Input: part model. Units: mm. Frame: model coordinates. Face numbers are marked on the shaded views. A direction names the side the tool comes from. Coordinates: 2 decimals unless noted, no trailing zeros. Order: outer loops, then holes, each group sorted by start corner. A loop starts at its lowest first (then second) coordinate and runs counter-clockwise, first axis right, second up. Notation, with made-up numbers: (55.5, 32) -> (97.5, 32) arc R18 cw to (97.5, 54) -> close; hole circle Ø10 at (84.5, 40). An arc over 180 degrees is marked (long way). One line per item, written item: value. Start each with the question number.
from build123d import *

# Parameters (mm, degrees)
SKETCH_1_R               = 6
SKETCH_1_R_2             = 2
EXTRUDE_1_DEPTH          = 2
SKETCH_2_R               = 1
CUT_EXTRUDE_8_DEPTH      = 40.131189606
PATTERN_CIRCULAR_2_COUNT = 4


with BuildPart() as part:
    # 草图1 → 凸台-拉伸1 (new body)
    with BuildSketch(Plane.XY):
        with BuildLine():
            Line((-3.413784582, 34.772058824), (-10.729037258, 2.426470588))
            ThreePointArc((-10.729037258, 2.426470588), (0, -11), (10.729037258, 2.426470588))
            Line((10.729037258, 2.426470588), (3.413784582, 34.772058824))
            ThreePointArc((3.413784582, 34.772058824), (0, 37.5), (-3.413784582, 34.772058824))
        make_face()
        Circle(SKETCH_1_R, mode=Mode.SUBTRACT)
        with Locations((0, 34)):
            Circle(SKETCH_1_R_2, mode=Mode.SUBTRACT)
        with BuildLine():
            Line((-2.989565186, 26.25), (-3.986086914, 14.333333333))
            ThreePointArc((-3.986086914, 14.333333333), (0, 10), (3.986086914, 14.333333333))
            Line((3.986086914, 14.333333333), (2.989565186, 26.25))
            ThreePointArc((2.989565186, 26.25), (0, 29), (-2.989565186, 26.25))
        make_face(mode=Mode.SUBTRACT)
    extrude(amount=EXTRUDE_1_DEPTH)

    # 草图2 → 切除-拉伸8 (cut, through all)
    with BuildSketch(Plane.XY):
        with Locations((6.01040764, -6.01040764)):
            Circle(SKETCH_2_R)
    cut_extrude_8 = extrude(amount=CUT_EXTRUDE_8_DEPTH, mode=Mode.SUBTRACT)

    # 阵列(圆周)2: 切除-拉伸8 ×4 about axis
    pattern_circular_2_axis = Axis((0, 0, 0), (0, 0, 1))
    for i in range(1, PATTERN_CIRCULAR_2_COUNT):
        add(cut_extrude_8.rotate(pattern_circular_2_axis, i * 360 / PATTERN_CIRCULAR_2_COUNT), mode=Mode.SUBTRACT)


solid = part.part
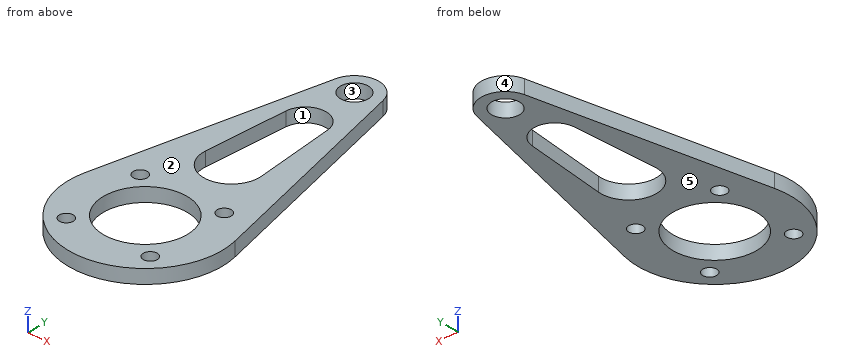
1) Pin query (flat end, axial travel): pin 1 Ø1 at (y, z) = (18, 1.5) entering from +X. Return the tip coordinate at first contact, or that it passes through.
2) Section query C-C, the plane z = 1.3. Return the cut outline in (x, y), plus the area to 3 significant figures.
3) Section query A-A, the plane x = 0. Return the cut outline in (y, z), plus the area to 3 significant figures.
4) Mould query, pull axis Y, two halves, no side actions, for the marked faces 3, 4 and 5. Classes: +Y half, -Y half, draft (parallel to the pull), parting line (faces both ways), or undercut.
5) Section query B-B, the plane y = 0. Return the cut outline in (x, z), plus the area to 3 significant figures.
6) Section query D-D, the plane x = 4.5. Return the cut outline in (y, z).
7) Ray query, line 1 along Y through (x, z) = (0.25, 0.85); line 2 along Y through (x, z) = (-1, 1.65); line 3 along X through (y, z) = (3, 1.6). Return the intervals inside material, ascending. Write a range as from..to.
8) Access query for the marked faces 1 and 2. Directions: +Z, -Z, +X, -X, +Y, -Y. A direction counts if a zero-diameter tool reaches every point of the face in a straight line with its end or side. Return the directions, or none.
Entries:
1. pin 1: stops at x = 7.32
2. outline: (-10.73, 2.43) arc R11 ccw (long way) to (10.73, 2.43) -> (3.41, 34.77) arc R3.5 ccw to (-3.41, 34.77) -> close; hole circle Ø2 at (-6.01, -6.01); hole circle Ø2 at (-6.01, 6.01); hole circle Ø12 at (0, 0); hole (-3.99, 14.33) arc R4 ccw (long way) to (3.99, 14.33) -> (2.99, 26.25) arc R3 ccw to (-2.99, 26.25) -> close; hole circle Ø4 at (0, 34); hole circle Ø2 at (6.01, -6.01); hole circle Ø2 at (6.01, 6.01)
2. area: 453 mm2
3. outline: (-11, 0) -> (-6, 0) -> (-6, 2) -> (-11, 2) -> close; (6, 0) -> (10, 0) -> (10, 2) -> (6, 2) -> close; (29, 0) -> (32, 0) -> (32, 2) -> (29, 2) -> close; (36, 0) -> (37.5, 0) -> (37.5, 2) -> (36, 2) -> close
3. area: 27.0 mm2
4. face 3: undercut
4. face 4: +Y half
4. face 5: draft
5. outline: (-11, 0) -> (-6, 0) -> (-6, 2) -> (-11, 2) -> close; (6, 0) -> (11, 0) -> (11, 2) -> (6, 2) -> close
5. area: 20.0 mm2
6. outline: (-10.04, 0) -> (-3.97, 0) -> (-3.97, 2) -> (-10.04, 2) -> close; (3.97, 0) -> (29.97, 0) -> (29.97, 2) -> (3.97, 2) -> close
7. line 1: y = -11..-5.99, 5.99..10.01, 28.99..32.02, 35.98..37.49
7. line 2: y = -10.95..-5.92, 5.92..10.13, 28.83..32.27, 35.73..37.35
7. line 3: x = -10.6..-5.2, 5.2..10.6
8. face 1: +Z, -Z
8. face 2: +Z, +X, -X, +Y, -Y
